Part print with two shaded views. Sizes in mm from the minimum x, y, z corner. A direction names the side the tool comes from. Coordinates: 2 decimals unless noted, no trailing zeros. Order: outer loops, then holes, each group sorted by start corner. A loop starts at its lowest first (then second) coordinate and runs counter-clockwise, first axis right, second up.
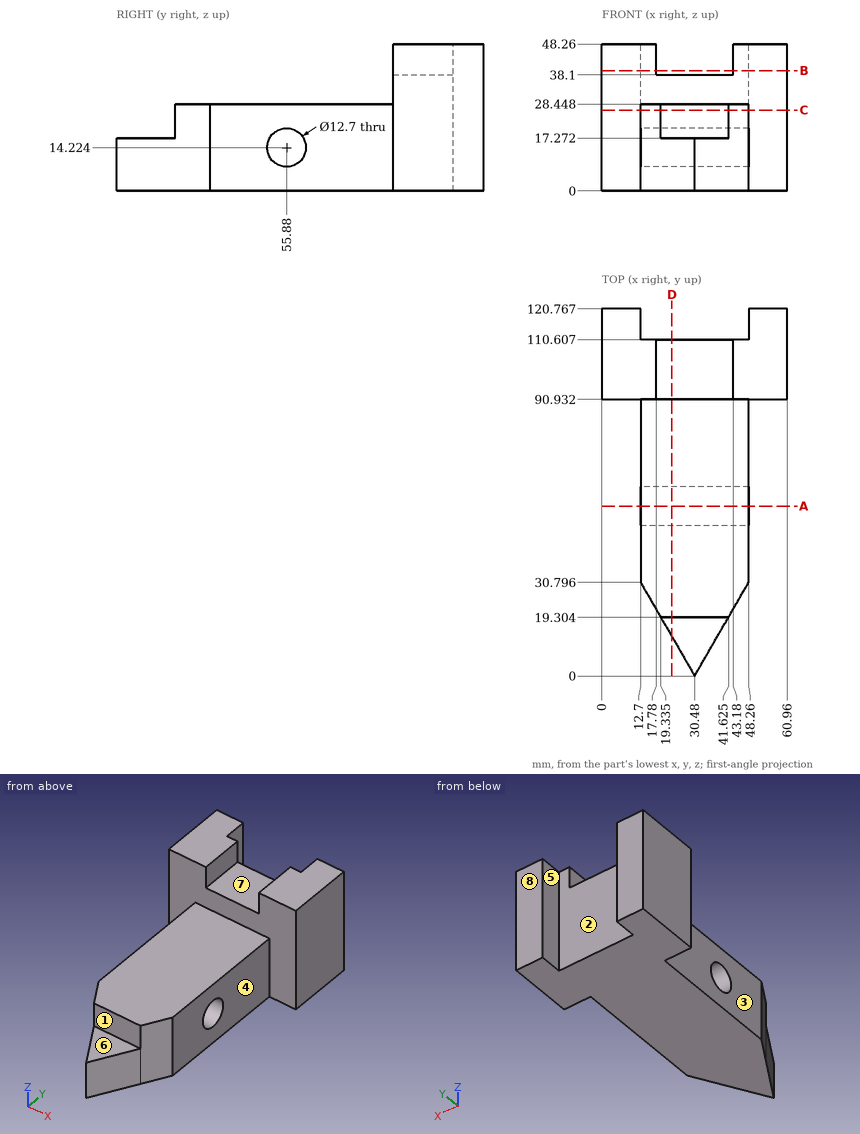
Q1. Cut at D-D on x = 23. Write the cut outline in (y, z), and give its area (3 significant figures).
Results list:
outline: (12.96, 0) - (110.61, 0) - (110.61, 38.1) - (90.93, 38.1) - (90.93, 28.45) - (19.3, 28.45) - (19.3, 17.27) - (12.96, 17.27) - close; hole circle Ø12.7 at (55.88, 14.22)
area: 2,770 mm2
Q2. Mould opens along X. For the marked faces 1, 2 and 3 say: pulls with the +X half, pulls with the -X half, needs draft (parallel to the pull), parting line crosses it, or undercut.
Results list:
face 1: needs draft
face 2: undercut
face 3: pulls with the -X half
Q3. Cut at B-B on z = 39.5. Write the cut outline in (x, y).
Results list:
outline: (0, 90.93) - (17.78, 90.93) - (17.78, 110.61) - (12.7, 110.61) - (12.7, 120.77) - (0, 120.77) - close; (43.18, 90.93) - (60.96, 90.93) - (60.96, 120.77) - (48.26, 120.77) - (48.26, 110.61) - (43.18, 110.61) - close
Q4. Wall check: line 1 along X through (y, z) = (115, 5); line 2 along Z through (x, y) = (39, 55.88); line 3 along Y through (x, z) = (12, 3). Give the ranges that are in metal, low to high.
Results list:
line 1: x = 0 to 12.7, 48.26 to 60.96
line 2: z = 0 to 7.87, 20.57 to 28.45
line 3: y = 90.93 to 120.77
Q5. Cut at C-C on z = 26.5. Write the cut outline in (x, y) (1 decimal).
Results list:
outline: (0, 90.9) - (12.7, 90.9) - (12.7, 30.8) - (19.3, 19.3) - (41.6, 19.3) - (48.3, 30.8) - (48.3, 90.9) - (61, 90.9) - (61, 120.8) - (48.3, 120.8) - (48.3, 110.6) - (12.7, 110.6) - (12.7, 120.8) - (0, 120.8) - close
Q6. Pin check, flat tips, straight feed: pin 1 Ø11.5 at (y, z) = (55.88, 14.224) entering from -X; pin 2 Ø4 at (x, y) = (23.5, 74.5) entering from +Z; pin 3 Ø14 at (y, z) = (69, 13) entering from -X; pin 4 Ø5 at (y, z) = (52, 26.5) entering from +X. Stop position of each tip, or through.
Results list:
pin 1: passes through
pin 2: stops at z = 28.45
pin 3: stops at x = 12.7
pin 4: stops at x = 48.26
Q7. Cut at A-A on y = 55.88. Write the cut outline in (x, z).
Results list:
outline: (12.7, 0) - (48.26, 0) - (48.26, 7.87) - (12.7, 7.87) - close; (12.7, 20.57) - (48.26, 20.57) - (48.26, 28.45) - (12.7, 28.45) - close
Q8. Which spindle directions (+Z, -Z, +X, -X, +Y, -Y) get a long thin tool onto all of the face, cutting with end or side? Do the marked faces 4, 5, 6, 7 and 8. Say none if no direction does.
Results list:
face 4: +Z, -Z, +X, -Y
face 5: +Z, -Z, +Y
face 6: +Z, +X, -X, -Y
face 7: +Z, +Y, -Y
face 8: +Z, -Z, +X, -X, +Y
